```python
from build123d import *

# Parameters (mm, degrees)
PAD003_DEPTH    = 25
SKETCH009_R     = 1.375
POCKET005_DEPTH = 7
SKETCH010_R     = 2.25
POCKET006_DEPTH = 5
FILLET011_R     = 1
CHAMFER_SIZE    = 1


with BuildPart() as part:
    # Sketch007 (on XY_Plane002 of Origin004) → Pad003 (new body)
    with BuildSketch(Plane.XY):
        with BuildLine():
            ThreePointArc((0, -9.5), (9.5, 0), (0, 9.5))
            Line((0, 9.5), (0, 10.356158))
            Line((0, 20.356158), (0, 10.356158))
            Line((5, 20.356158), (0, 20.356158))
            Line((5, 10.356158), (5, 20.356158))
            ThreePointArc((6.480515, -9.500154), (11.468166, 0.855083), (5, 10.356158))
            Line((15, -9.5), (6.480515, -9.500154))
            Line((15, -17), (15, -9.5))
            Line((0, -17), (15, -17))
            Line((0, -9.5), (0, -17))
        make_face()
    extrude(amount=PAD003_DEPTH)

    # Sketch009 (on Face3 of Pad003) → Pocket005 (cut)
    with BuildSketch(Plane.XZ.offset(17)):
        with Locations((7.5, 12.5)):
            Circle(SKETCH009_R)
    extrude(amount=-POCKET005_DEPTH, mode=Mode.SUBTRACT)

    # Sketch010 (on Face10 of Pocket005) → Pocket006 (cut)
    with BuildSketch(Plane.YZ.offset(5)):
        with Locations((15.356158, 12.5)):
            Circle(SKETCH010_R)
    extrude(amount=-POCKET006_DEPTH, mode=Mode.SUBTRACT)

    # Fillet011
    fillet011_edges = [part.edges().sort_by_distance(p)[0] for p in [
        (15, -13.25, 0),
    ]]
    fillet(fillet011_edges, radius=FILLET011_R)

    # Chamfer
    chamfer_edges = [part.edges().sort_by_distance(p)[0] for p in [
        (6.125, -17, 12.5),
    ]]
    chamfer(chamfer_edges, length=CHAMFER_SIZE)


solid = part.part
```
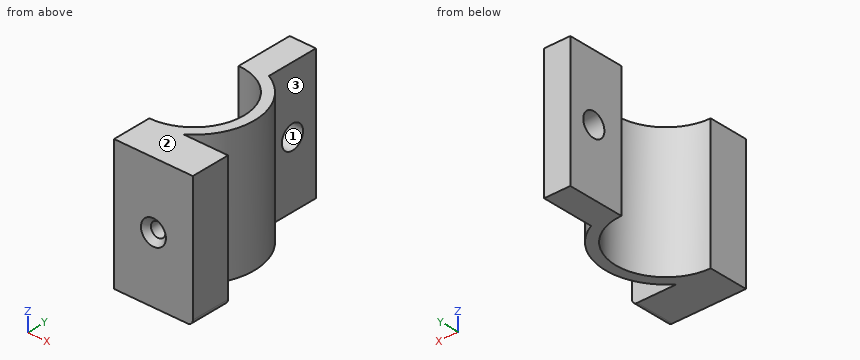
Check sheet for the modelled part. Datum: model origin and axes. Units: mm. Face numbers are marked on the shaded views. Give positions to 0.01 mm unless a question says otherwise; leave off trailing zeros. Loops run counter-clockwise (first coordinate to the right, second up) from the corner with the lowest first, then second, coordinate; pieces in that order, holes last. Notation, with made-up numbers: (-39, -32) - (-18, -32) arc R30 ccw to (-18, -5) - close; hole circle Ø5 at (84, 56.5). An arc over 180 degrees is marked (long way). One line per question, with ' | ' between items. Start each with the question number.
1. Cross-section at C-C, the plane y = -12. Enter the section's corners in (x, z) (3 decimals).
2. Cross-section at A-A, the plane x = 4.25. Enter the section's corners in (y, z), plus the area to 3 significant figures.
3. Cross-section at D-D, the plane y = 13.5. Enter the section's corners in (x, z).
4. Gauge pin test, flat ends, axial feed: pin 1 Ø11 at (y, z) = (14, 11) entering from +X; pin 2 Ø2 at (y, z) = (-4, 22.5) entering from -X; pin 3 Ø3 at (x, z) = (7.5, 12.5) entering from -Y (3 decimals). Record the tip position at first contact, or that the pin passes through.
5. Draft check along Z on the marked faces 1, 2 and 3. Enter one of: released by +Z, released by -Z, zero draft, split by the parting line, or undercut.
6. Material ranges on line 1 along Z through (x, y) = (7.5, -12.15) (3 decimals); line 2 along Y through (x, z) = (8.5, 10.5); line 3 along X through (y, z) = (13, 8.75), recorded low to high. Write a range as [from, to].
7. Cross-section at B-B, the plane z = 12.5. Enter the section's corners in (x, y) (3 decimals), plus the area to 3 significant figures.
Check result:
1) outline: (0, 0) - (14, 0) arc R1 ccw to (15, 1) - (15, 25) - (0, 25) - close; hole circle Ø2.75 at (7.5, 12.5)
2) outline: (-17, 0) - (-8.5, 0) - (-8.5, 25) - (-17, 25) - close; (8.5, 0) - (20.36, 0) - (20.36, 25) - (8.5, 25) - close; hole circle Ø4.5 at (15.36, 12.5) | area: 493 mm2
3) outline: (0, 0) - (5, 0) - (5, 11.23) - (0, 11.23) - close; (0, 13.77) - (5, 13.77) - (5, 25) - (0, 25) - close
4) pin 1: stops at x = 7.75 | pin 2: stops at x = 8.08 | pin 3: stops at y = -16.125
5) face 1: undercut | face 2: released by +Z | face 3: zero draft
6) line 1: z = [0, 11.125], [13.875, 25] | line 2: y = [-16.86, -9.5], [-7.75, -4.24], [4.24, 7.75] | line 3: x = [0, 5]
7) outline: (0, -17) - (5.125, -17) - (6.125, -16) - (6.125, -10) - (8.875, -10) - (8.875, -16) - (9.875, -17) - (15, -17) - (15, -9.5) - (6.481, -9.5) arc R11.5 ccw to (5, 10.356) - (5, 13.106) - (0, 13.106) - (0, 9.5) arc R9.5 cw to (0, -9.5) - close; (0, 17.606) - (5, 17.606) - (5, 20.356) - (0, 20.356) - close | area: 173 mm2
